Source: CAD feature listing. Evaluate the final solid. Frame: model axes, mm. Round coordinates to 2 decimals unless told otherwise and drop trailing zeros. Order: outer loops, then holes, each group sorted by start corner. A loop starts at its lowest first (then second) coordinate and runs counter-clockwise, first axis right, second up. Notation, with made-up numbers: (75.25, 49) -> (110.25, 49) arc R21 ccw to (110.25, 73) -> close; hole circle Ø8 at (55, 41). An arc over 180 degrees is marked (long way). Write item = value, one per line. Start each with the question number.
(1) Ray query, line 1 (Y direction, x = 10, z = 4.05); line 2 (X direction, y = 3.5, z = 3.3); line 3 (Y direction, x = -13.5, z = 1.25). Return the intervals inside material, ascending.
(2) Cut plane A-A on x = 10. Return the cut outline in (y, z).
(3) Cut plane D-D on x = 6.5. Return the cut outline in (y, z).
(4) Cut plane B-B on y = 0. Return the cut outline in (x, z).
(5) Contact query for a flat-ended pin moving along its axis: pin 1 Ø7 at (x, y) = (-10, 0) entering from +Z (3 decimals). Output: stop coordinate, or through.
(6) Draft query along X for faces 1 (the face through (-17.5, 0, 3)), 2 (the face through (0, 0, 0)), 3 (the face through (-13.2, -2.4, 3)), 4 (the face through (17.5, 0, 3)). Return one class per face: released by +X, released by -X, zero draft, split by the parting line, or undercut.
(7) Cut plane C-C on z = 4.85. Return the cut outline in (x, y), then the cut area to 3 significant figures.
from build123d import *

# Parameters (mm, degrees)
SKETCH1_W           = 35
SKETCH1_H           = 50
SKETCH1_R           = 4
BOSS_EXTRUDE1_DEPTH = 6
FILLET1_R           = 0.5


with BuildPart() as part:
    # Sketch1 → Boss-Extrude1 (new body)
    with BuildSketch(Plane.XY):
        Rectangle(SKETCH1_W, SKETCH1_H)
        with Locations((-10, 0)):
            Circle(SKETCH1_R, mode=Mode.SUBTRACT)
        with Locations((10, 0)):
            Circle(SKETCH1_R, mode=Mode.SUBTRACT)
    extrude(amount=BOSS_EXTRUDE1_DEPTH)

    # Fillet1
    fillet1_edges = [part.edges().sort_by_distance(p)[0] for p in [
        (-17.5, 0, 6),
        (0, -25, 6),
        (17.5, 0, 6),
        (0, -25, 0),
        (-17.5, 0, 0),
        (0, 25, 0),
        (17.5, 0, 0),
        (17.5, -25, 3),
        (-17.5, -25, 3),
        (-17.5, 25, 3),
        (17.5, 25, 3),
        (0, 25, 6),
    ]]
    fillet(fillet1_edges, radius=FILLET1_R)


solid = part.part
Evaluation:
q1.line_1 = -25 to -4, 4 to 25
q1.line_2 = -17.5 to -11.94, -8.06 to 8.06, 11.94 to 17.5
q1.line_3 = -25 to -1.94, 1.94 to 25
q2.outline = (-25, 0.5) arc R0.5 ccw to (-24.5, 0) -> (-4, 0) -> (-4, 6) -> (-24.5, 6) arc R0.5 ccw to (-25, 5.5) -> close; (4, 0) -> (24.5, 0) arc R0.5 ccw to (25, 0.5) -> (25, 5.5) arc R0.5 ccw to (24.5, 6) -> (4, 6) -> close
q3.outline = (-25, 0.5) arc R0.5 ccw to (-24.5, 0) -> (-1.94, 0) -> (-1.94, 6) -> (-24.5, 6) arc R0.5 ccw to (-25, 5.5) -> close; (1.94, 0) -> (24.5, 0) arc R0.5 ccw to (25, 0.5) -> (25, 5.5) arc R0.5 ccw to (24.5, 6) -> (1.94, 6) -> close
q4.outline = (-17.5, 0.5) arc R0.5 ccw to (-17, 0) -> (-14, 0) -> (-14, 6) -> (-17, 6) arc R0.5 ccw to (-17.5, 5.5) -> close; (-6, 0) -> (6, 0) -> (6, 6) -> (-6, 6) -> close; (14, 0) -> (17, 0) arc R0.5 ccw to (17.5, 0.5) -> (17.5, 5.5) arc R0.5 ccw to (17, 6) -> (14, 6) -> close
q5.pin_1 = through
q6.face_1 = released by -X
q6.face_2 = zero draft
q6.face_3 = undercut
q6.face_4 = released by +X
q7.outline = (-17.5, -24.5) arc R0.5 ccw to (-17, -25) -> (17, -25) arc R0.5 ccw to (17.5, -24.5) -> (17.5, 24.5) arc R0.5 ccw to (17, 25) -> (-17, 25) arc R0.5 ccw to (-17.5, 24.5) -> close; hole circle Ø8 at (-10, 0); hole circle Ø8 at (10, 0)
q7.area = 1,650 mm^2
